```python
from build123d import *

# Parameters (mm, degrees)
F1_DEPTH = 12
F2_R     = 2
F3_R     = 3
F4_DEPTH = 50


with BuildPart() as f1:
    # F0 (on Top) → F1 (new body)
    with BuildSketch(Plane.XY):
        with BuildLine():
            Line((-0.5, 12), (-0.5, 4.974937))
            ThreePointArc((-0.5, 4.974937), (-3.535534, 3.535534), (-4.974937, 0.5))
            Line((-4.974937, 0.5), (-12, 0.5))
            Line((-12, 0.5), (-12, -0.5))
            Line((-12, -0.5), (-4.974937, -0.5))
            ThreePointArc((-4.974937, -0.5), (-3.535534, -3.535534), (-0.5, -4.974937))
            Line((-0.5, -4.974937), (-0.5, -12))
            Line((-0.5, -12), (0.5, -12))
            Line((0.5, -12), (0.5, -4.974937))
            ThreePointArc((0.5, -4.974937), (3.535534, -3.535534), (4.974937, -0.5))
            Line((4.974937, -0.5), (12, -0.5))
            Line((12, -0.5), (12, 0.5))
            Line((12, 0.5), (4.974937, 0.5))
            ThreePointArc((4.974937, 0.5), (3.535534, 3.535534), (0.5, 4.974937))
            Line((0.5, 4.974937), (0.5, 12))
            Line((0.5, 12), (-0.5, 12))
        make_face()
    extrude(amount=F1_DEPTH)

    # F2
    f2_edges = [f1.edges().sort_by_distance(p)[0] for p in [
        (-12, 0, 12),
        (-12, 0, 0),
        (0, 12, 12),
        (12, 0, 12),
        (0, -12, 12),
        (0, 12, 0),
        (12, 0, 0),
        (0, -12, 0),
    ]]
    fillet(f2_edges, radius=F2_R)

    # F3 (on face) → F4 (join)
    with BuildSketch(Plane(origin=(0, 0, 0), x_dir=(1, 0, 0), z_dir=(0, 0, -1))):
        Circle(F3_R)
    extrude(amount=F4_DEPTH)


solid = f1.part
```
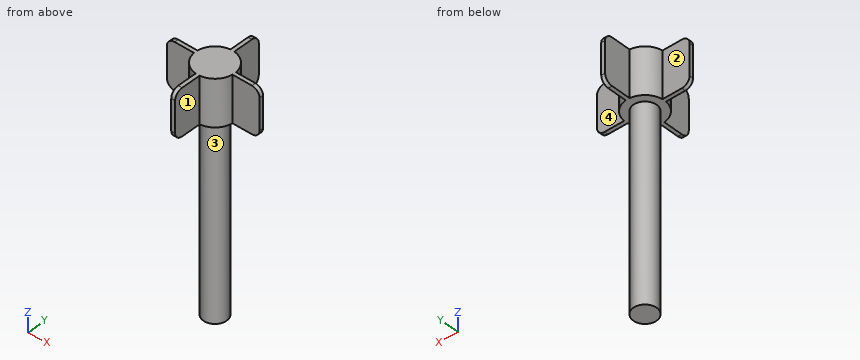
Source: CAD feature listing. Evaluate the final solid. Frame: model axes, mm. Face numbers are marked on the shaded views. A direction names the side the tool comes from. Round coordinates to 2 decimals unless told otherwise and drop trailing zeros. Write each loop counter-clockwise with the first axis right and the second up, starting at its lowest first coordinate (ties: lowest second). Pieces come first, ordered by that corner, then holes. Notation, with made-up numbers: M 38,34 L 43,34 A21 ccw 43,65 Z; hole C 49,86.25 d2. An arc over 180 degrees is marked long. Use CSV: the item, a comma, the result in double quotes. Start each with the question number.
Q1. First-contact query: P1, Ø7.5, axis at x = -8, z = 6, coming from the -Y side; P2, Ø5.5, axis at x = -8.5, z = 8.5, coming from the +Y side; P3, Ø6, axis at x = -1, y = -3, coming from the -Z side; P4, Ø5.5, axis at y = 9, z = 8.5, coming from the +X side. Flat tips, straight axial feed; report the tip coordinate or a pass-through.
Q2. Line query: line 1 (Z direction, x = 2, y = -2.75); line 2 (X direction, y = -4, z = 0.5); line 3 (X direction, y = -9.25, z = 3.5). Output: solid intervals per line, ascending. Write a range as from..to.
Q3. Cut plane B-B on x = 2. Output: boundary loops of the cut face in (y, z).
Q4. Access query for the marked faces 1, 2, 3 and 4. Directions: +Z, -Z, +X, -X, +Y, -Y. A direction counts if a zero-diameter tool reaches every point of the face in a straight line with its end or side. Return the directions, or none.
Q5. Cut plane A-A on z = 6.5. Output: boundary loops of the cut face in (x, y).
Q6. Cut plane C-C on y = -8.75. Output: boundary loops of the cut face in (x, z), plus the area to 3 significant figures.
Q7. Cut plane D-D on z = -38. Output: boundary loops of the cut face in (x, y), plus the area to 3 significant figures.
Results found:
1,P1,"y = -2.63"
1,P2,"y = 0.5"
1,P3,"z = -50"
1,P4,"x = 0.5"
2,line 1,"0..12"
2,line 2,"-3..3"
2,line 3,"-0.5..0.5"
3,outline,"M -4.58,0 L -2.24,0 L -2.24,-50 L 2.24,-50 L 2.24,0 L 4.58,0 L 4.58,12 L -4.58,12 Z"
4,face 1,"+Z, -Z, +X, -Y"
4,face 2,"+Z, -Z, -X, +Y"
4,face 3,"-Z"
4,face 4,"+Z, -Z, +X, +Y"
5,outline,"M -12,-0.5 L -4.97,-0.5 A5 ccw -0.5,-4.97 L -0.5,-12 L 0.5,-12 L 0.5,-4.97 A5 ccw 4.97,-0.5 L 12,-0.5 L 12,0.5 L 4.97,0.5 A5 ccw 0.5,4.97 L 0.5,12 L -0.5,12 L -0.5,4.97 A5 ccw -4.97,0.5 L -12,0.5 Z"
6,outline,"M -0.5,0 L 0.5,0 L 0.5,12 L -0.5,12 Z"
6,area,"12.0 mm^2"
7,outline,"C 0,0 d6"
7,area,"28.3 mm^2"
